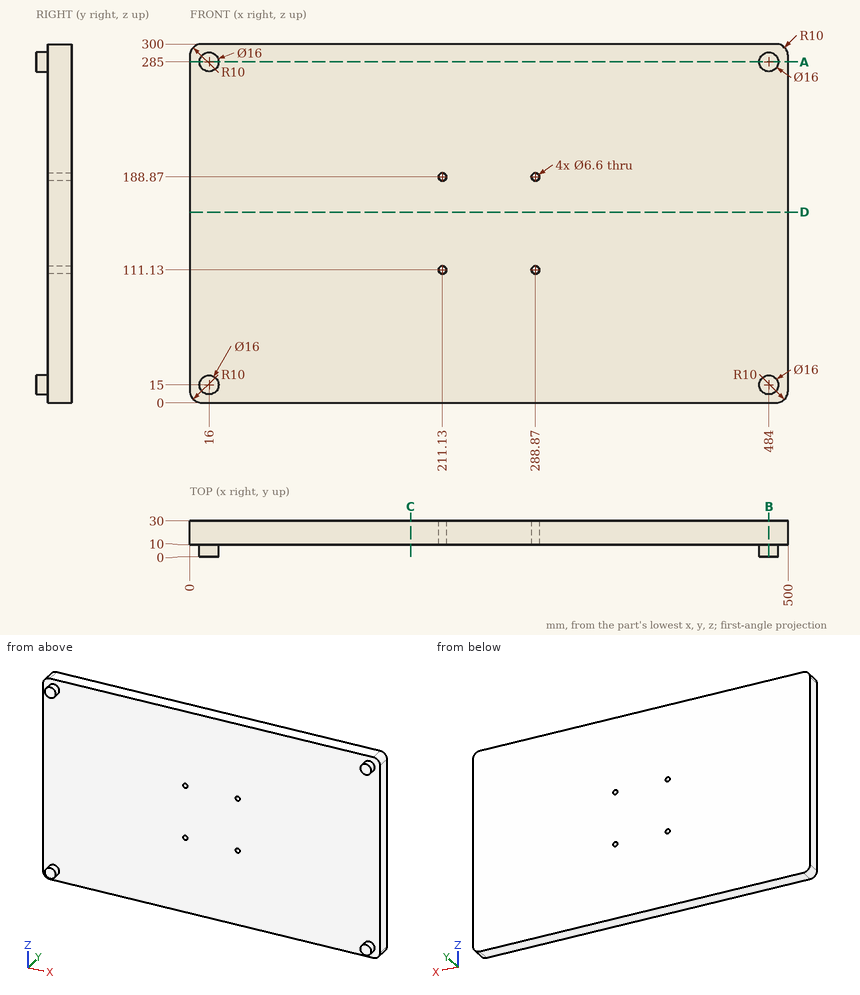
Could you check a few things on this drawing? It's one solid part, dimensions in mm from its lowest x, y, z. Coordinates: 2 decimals unless noted, no trailing zeros. Write each loop counter-clockwise with the first axis right and the second up, starting at its lowest first coordinate (ties: lowest second). Pieces come first, ordered by that corner, then holes. Notation, with made-up numbers: M -21.5,77 L 12.5,77 A26 cw 12.5,116 Z; hole C -24,-4.5 d7. An arc over 180 degrees is marked long. One line per question, with ' | ' between items.
1) Imagine slicing it at A-A, the plane z = 285. Write out the boundary of the cut face in (x, y), and give its area (3 significant figures).
Checks:
outline: M 0,10 L 8,10 L 8,0 L 24,0 L 24,10 L 476,10 L 476,0 L 492,0 L 492,10 L 500,10 L 500,30 L 0,30 Z | area: 10,300 mm²
2) Imagine slicing it at B-B, the plane x = 484. Write out the boundary of the cut face in (y, z), and give its area (3 significant figures).
Checks:
outline: M 0,7 L 10,7 L 10,0 L 30,0 L 30,300 L 10,300 L 10,293 L 0,293 L 0,277 L 10,277 L 10,23 L 0,23 Z | area: 6,320 mm²
3) Imagine slicing it at C-C, the plane x = 184.5. Write out the boundary of the cut face in (y, z).
Checks:
outline: M 10,0 L 30,0 L 30,300 L 10,300 Z
4) For pin 1 Ø10 at (x, y) = (306.5, 20.5) entering from -Z; pin 2 Ø8.5 at (x, z) = (211.13, 188.87) entering from -Y, each with a flat end and sliding along its axis, tell me the tip position at first contact or that it passes through.
Checks:
pin 1: z = 0 | pin 2: y = 10
5) I need wall thicknesses on probe 1 along X at (y, z) = (15.5, 111.13); probe 2 along Z at (x, y) = (211.13, 19.5); probe 3 along Z at (x, y) = (291.5, 15.5). Which ranges of each line are inside material? Lowest first, please. Write a range as [from, to].
Checks:
probe 1: [0, 207.83], [214.43, 285.57], [292.17, 500] | probe 2: [0, 107.83], [114.43, 185.57], [192.17, 300] | probe 3: [0, 109.14], [113.12, 186.88], [190.86, 300]
6) Imagine slicing it at D-D, the plane z = 159.5. Write out the boundary of the cut face in (x, y), and give its area (3 significant figures).
Checks:
outline: M 0,10 L 500,10 L 500,30 L 0,30 Z | area: 10,000 mm²
